```python
from build123d import *

# Parameters (mm, degrees)
F0_W     = 400
F0_H     = 400
F0_R     = 5.5
F0_W_2   = 300
F0_H_2   = 300
F1_DEPTH = 5


with BuildPart() as f1:
    # F0 (on Top) → F1 (new body)
    with BuildSketch(Plane.XY):
        Rectangle(F0_W, F0_H)
        with Locations((-175, -175)):
            Circle(F0_R, mode=Mode.SUBTRACT)
        with Locations((-87.5, -175)):
            Circle(F0_R, mode=Mode.SUBTRACT)
        with Locations((-175, -87.5)):
            Circle(F0_R, mode=Mode.SUBTRACT)
        with Locations((0, -175)):
            Circle(F0_R, mode=Mode.SUBTRACT)
        with Locations((87.5, -175)):
            Circle(F0_R, mode=Mode.SUBTRACT)
        with Locations((175, -175)):
            Circle(F0_R, mode=Mode.SUBTRACT)
        with Locations((175, -87.5)):
            Circle(F0_R, mode=Mode.SUBTRACT)
        with Locations((-175, 0)):
            Circle(F0_R, mode=Mode.SUBTRACT)
        with Locations((-175, 87.5)):
            Circle(F0_R, mode=Mode.SUBTRACT)
        with Locations((-175, 175)):
            Circle(F0_R, mode=Mode.SUBTRACT)
        with Locations((-87.5, 175)):
            Circle(F0_R, mode=Mode.SUBTRACT)
        Rectangle(F0_W_2, F0_H_2, mode=Mode.SUBTRACT)
        with Locations((175, 0)):
            Circle(F0_R, mode=Mode.SUBTRACT)
        with Locations((175, 87.5)):
            Circle(F0_R, mode=Mode.SUBTRACT)
        with Locations((0, 175)):
            Circle(F0_R, mode=Mode.SUBTRACT)
        with Locations((87.5, 175)):
            Circle(F0_R, mode=Mode.SUBTRACT)
        with Locations((175, 175)):
            Circle(F0_R, mode=Mode.SUBTRACT)
    extrude(amount=F1_DEPTH)


solid = f1.part
```
Geometry check sheet. Reference: the model listing, model coordinates, mm. Coordinates: 2 decimals unless noted, no trailing zeros. Loops run counter-clockwise (first coordinate to the right, second up) from the corner with the lowest first, then second, coordinate; pieces in that order, holes last.
Item 1: Release check for a two-part mould opening along Y. For faces 1 (the face through (-1.19, -180.37, 2.46)), 2 (the face through (-164, 16, 5)) record: released by +Y, released by -Y, zero draft, split by the parting line, or undercut.
Item 2: Go/stop test with a flat-tipped pin: pin 1 Ø17.5 at (x, y) = (-175, 175) entering from +Z. Record where the tip stops, or that it passes through.
Item 3: Sectioned sample at A-A, the plane x = 108. Record the boundary of the cut face in (y, z).
Item 4: Sectioned sample at C-C, the plane z = 3.95. Count the separate pieces of the cut face and the enclosed holes in it, then the cut area to 3 significant figures.
Item 5: Thickness scan on line 1 (Y direction, x = -103, z = 4.1); line 2 (Y direction, x = -175, z = 1.8). Record the ranges inside material, lowest first.
Item 6: Sectioned sample at D-D, the plane y = 175. Record the boundary of the cut face in (x, z).
Check result:
1. face 1: undercut
1. face 2: zero draft
2. pin 1: stops at z = 5
3. outline: (-200, 0) - (-150, 0) - (-150, 5) - (-200, 5) - close; (150, 0) - (200, 0) - (200, 5) - (150, 5) - close
4. separate pieces: 1
4. enclosed holes: 17
4. area: 68,500 mm2
5. line 1: y = -200 to -150, 150 to 200
5. line 2: y = -200 to -180.5, -169.5 to -93, -82 to -5.5, 5.5 to 82, 93 to 169.5, 180.5 to 200
6. outline: (-200, 0) - (-180.5, 0) - (-180.5, 5) - (-200, 5) - close; (-169.5, 0) - (-93, 0) - (-93, 5) - (-169.5, 5) - close; (-82, 0) - (-5.5, 0) - (-5.5, 5) - (-82, 5) - close; (5.5, 0) - (82, 0) - (82, 5) - (5.5, 5) - close; (93, 0) - (169.5, 0) - (169.5, 5) - (93, 5) - close; (180.5, 0) - (200, 0) - (200, 5) - (180.5, 5) - close
